```python
from build123d import *

# Parameters (mm, degrees)
F0_R     = 1.5
F1_DEPTH = 3


with BuildPart() as f1:
    # F0 (on Top) → F1 (new body)
    with BuildSketch(Plane.XY):
        with BuildLine():
            Line((15.9, 6.05), (-15.9, 6.05))
            Line((-15.9, 6.05), (-15.9, 0.92558))
            Line((-15.9, 0.92558), (-15.180382, 0.92558))
            ThreePointArc((-15.180382, 0.92558), (-12.5, 0), (-15.180382, -0.92558))
            Line((-15.180382, -0.92558), (-15.9, -0.92558))
            Line((-15.9, -0.92558), (-15.9, -6.05))
            Line((-15.9, -6.05), (15.9, -6.05))
            Line((15.9, -6.05), (15.9, -0.92558))
            Line((15.9, -0.92558), (15.180382, -0.92558))
            ThreePointArc((15.180382, -0.92558), (12.5, 0), (15.180382, 0.92558))
            Line((15.180382, 0.92558), (15.9, 0.92558))
            Line((15.9, 0.92558), (15.9, 6.05))
        make_face()
        with Locations((-5.88706, 0)):
            Circle(F0_R, mode=Mode.SUBTRACT)
    extrude(amount=F1_DEPTH)


solid = f1.part
```
Could you check a few things on this model? Use its own coordinates, in mm. Round coordinates to 2 decimals unless told otherwise and drop trailing zeros. Loops run counter-clockwise (first coordinate to the right, second up) from the corner with the lowest first, then second, coordinate; pieces in that order, holes last. Notation, with made-up numbers: (60, 62) -> (109, 62) arc R19 ccw to (109, 73) -> close; hole circle Ø4 at (83.25, 56). An arc over 180 degrees is marked (long way). Put each result on its own line as item: value.
Q1. Thinking about a two-plate mould opening in X: for faces 1 (the cylindrical face through (-12.5, 0.05, 1.48)), 2 (the flat face through (0, 0, 0)), 3 (the flat face through (15.9, -4, 1)), which applies, pulls with the +X half, pulls with the -X half, needs draft (parallel to the pull), parting line crosses it, or undercut?
Checks:
face 1: undercut
face 2: needs draft
face 3: pulls with the +X half
Q2. I want a section at A-A on y = 0. Write out the boundary of the cut face in (x, z).
Checks:
outline: (-12.5, 0) -> (-7.39, 0) -> (-7.39, 3) -> (-12.5, 3) -> close; (-4.39, 0) -> (12.5, 0) -> (12.5, 3) -> (-4.39, 3) -> close
Q3. I want a section at B-B on z = 0.85. Write out the boundary of the cut face in (x, y).
Checks:
outline: (-15.9, -6.05) -> (15.9, -6.05) -> (15.9, -0.93) -> (15.18, -0.93) arc R1.5 cw (long way) to (15.18, 0.93) -> (15.9, 0.93) -> (15.9, 6.05) -> (-15.9, 6.05) -> (-15.9, 0.93) -> (-15.18, 0.93) arc R1.5 cw (long way) to (-15.18, -0.93) -> (-15.9, -0.93) -> close; hole circle Ø3 at (-5.89, 0)
Q4. I want a section at C-C on x = -14. Write out the boundary of the cut face in (y, z).
Checks:
outline: (-6.05, 0) -> (-1.5, 0) -> (-1.5, 3) -> (-6.05, 3) -> close; (1.5, 0) -> (6.05, 0) -> (6.05, 3) -> (1.5, 3) -> close
Q5. Please list where these lines run through material, in increasing order: line 1 (Y direction, x = -14, z = 1.45); line 2 (X direction, y = -1, z = 1.1); line 3 (X direction, y = -1.25, z = 2.3). Write a range as from..to.
Checks:
line 1: -6.05..-1.5, 1.5..6.05
line 2: -15.9..-15.12, -12.88..-7.01, -4.77..12.88, 15.12..15.9
line 3: -15.9..-14.83, -13.17..-6.72, -5.06..13.17, 14.83..15.9
Q6. For pin 1 Ø1.8 at (x, y) = (14, 0) entering from -Z, with a flat end and sliding along its axis, tell me the tip position at first contact or that it passes through.
Checks:
pin 1: through
